Check sheet for the modelled part. Datum: model origin and axes. Units: mm. Face numbers are marked on the shaded views. A direction names the side the tool comes from. Round coordinates to 2 decimals unless told otherwise and drop trailing zeros. Loops run counter-clockwise (first coordinate to the right, second up) from the corner with the lowest first, then second, coordinate; pieces in that order, holes last. Notation, with made-up numbers: (20, -16.75) -> (46, -16.75) arc R32 cw to (46, 15.25) -> close; hole circle Ø3 at (22, -39). An arc over 180 degrees is marked (long way). One line per item, written item: value. Start each with the question number.
1. Release check for a two-part mould opening along X. For the marked faces 4, 5 and 6 record: +X half, -X half, draft (parallel to the pull), parting line (faces both ways), or undercut.
2. Material ranges on L1, parallel to Z at x = 0, y = 7.75; L2, parallel to X at y = 9, z = -22; L3, parallel to X at y = 5, z = 0, recorded low to high.
3. Cross-section at C-C on z = 19.5. Record the cut outline in (x, y), then the cut area to 3 significant figures.
4. Cross-section at A-A on x = 0. Record the cut outline in (y, z).
5. Cross-section at B-B on z = 0. Record the cut outline in (x, y).
6. Cross-section at D-D on x = 88. Record the cut outline in (y, z).
7. Go/stop test with flat-tipped pins: pin 1 (2.5 mm diameter, centred on y = 5.5, z = -21, fed in from -X); pin 2 (3 mm diameter, centred on x = 95, y = 5.5, fed in from +Z); pin 3 (6 mm diameter, centred on x = 31, y = 6.5, fed in from -Z). Record where each tip stops, or that it passes through.
8. Set-up check for the marked faces 1, 2 and 3: record each of +Z, -Z, +X, -X, +Y, -Y from which the full face is reachable in a straight line by a thin tool's end or side.
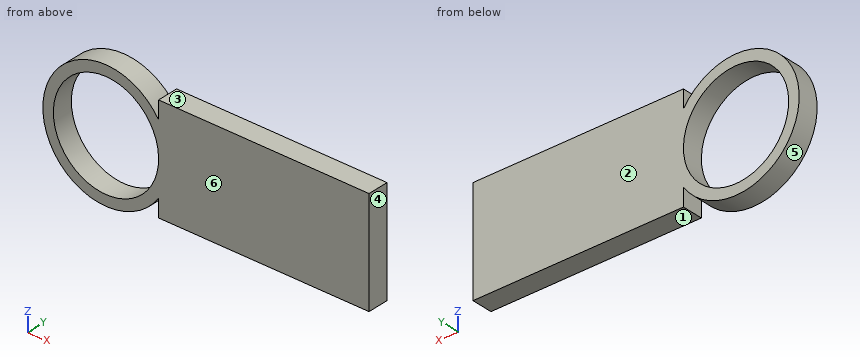
from build123d import *

# Parameters (mm, degrees)
SKETCH1_R           = 30
SKETCH1_R_2         = 25
BOSS_EXTRUDE1_DEPTH = 10
SKETCH3_W           = 100
SKETCH3_H           = 50
BOSS_EXTRUDE2_DEPTH = 10


with BuildPart() as part:
    # Sketch1 → Boss-Extrude1 (new body)
    with BuildSketch(Plane(origin=(0, 0, 0), x_dir=(1, 0, 0), z_dir=(0, 1, 0))):
        with Locations(Location((0, 0, 0), (0, 0, 270))):
            Circle(SKETCH1_R)
        with Locations(Location((0, 0, 0), (0, 0, 270))):
            Circle(SKETCH1_R_2, mode=Mode.SUBTRACT)
    extrude(amount=BOSS_EXTRUDE1_DEPTH)

    # Sketch3 → Boss-Extrude2 (add)
    with BuildSketch(Plane(origin=(0, 0, 0), x_dir=(1, 0, 0), z_dir=(0, 1, 0))):
        with Locations((75, 0)):
            Rectangle(SKETCH3_W, SKETCH3_H)
    extrude(amount=BOSS_EXTRUDE2_DEPTH)


solid = part.part
Taken from the geometry:
1. face 4: +X half
1. face 5: undercut
1. face 6: draft
2. L1: z = -30 to -25, 25 to 30
2. L2: x = -20.4 to -11.87, 11.87 to 20.4, 25 to 125
2. L3: x = -30 to -25, 25 to 125
3. outline: (-22.8, 0) -> (-15.64, 0) -> (-15.64, 10) -> (-22.8, 10) -> close; (15.64, 0) -> (22.8, 0) -> (22.8, 10) -> (15.64, 10) -> close; (25, 0) -> (125, 0) -> (125, 10) -> (25, 10) -> close
3. area: 1,140 mm2
4. outline: (0, -30) -> (10, -30) -> (10, -25) -> (0, -25) -> close; (0, 25) -> (10, 25) -> (10, 30) -> (0, 30) -> close
5. outline: (-30, 0) -> (-25, 0) -> (-25, 10) -> (-30, 10) -> close; (25, 0) -> (125, 0) -> (125, 10) -> (25, 10) -> close
6. outline: (0, -25) -> (10, -25) -> (10, 25) -> (0, 25) -> close
7. pin 1: stops at x = -22.58
7. pin 2: stops at z = 25
7. pin 3: stops at z = -25
8. face 1: -Z, +X, +Y, -Y
8. face 2: +Z, -Z, +X, -X, +Y
8. face 3: +Z, +X, +Y, -Y
